from build123d import *

# Parameters (mm, degrees)
SKETCH1_R               = 30
BOSS_EXTRUDE1_DEPTH     = 6
SKETCH2_R               = 14.5
BOSS_EXTRUDE2_DEPTH     = 13
CUT_EXTRUDE1_DEPTH      = 47.486557197
CUT_EXTRUDE1_DEPTH_BACK = 47.486557197
SKETCH3_R               = 12.75
BOSS_EXTRUDE4_START     = 13
SKETCH5_R               = 30
SKETCH5_R_2             = 12.75
BOSS_EXTRUDE4_DEPTH     = 6
CUT_EXTRUDE2_DEPTH      = 45.373415465
CUT_EXTRUDE2_DEPTH_BACK = 45.373415465
SKETCH6_R               = 2
CUT_EXTRUDE3_DEPTH      = 47.486557197
CUT_EXTRUDE3_DEPTH_BACK = 47.486557197
FILLET1_R               = 2
FILLET2_R               = 2
FILLET3_R               = 2
FILLET4_R               = 2
SKETCH8_R               = 4
BOSS_EXTRUDE5_DEPTH     = 13
FILLET5_R               = 2
FILLET6_R               = 2
FILLET7_R               = 2
FILLET8_R               = 2
CUT_EXTRUDE4_DEPTH      = 42.830642507
CUT_EXTRUDE4_DEPTH_BACK = 42.830642507
SKETCH11_W              = 25.5
SKETCH11_H              = 25


with BuildPart() as part:
    # Sketch1 → Boss-Extrude1 (new body)
    with BuildSketch(Plane.XY):
        Circle(SKETCH1_R)
    extrude(amount=-BOSS_EXTRUDE1_DEPTH)

    # Sketch2 → Boss-Extrude2 (add)
    with BuildSketch(Plane.XY):
        with Locations(Location((0, 0, 0), (0, 0, 180))):
            Circle(SKETCH2_R)
    extrude(amount=BOSS_EXTRUDE2_DEPTH)

    # Sketch3 → Cut-Extrude1 (cut, two sides: drawn at the far end of the back side and taken through both)
    with BuildSketch(Plane.XY.offset(13).offset(-CUT_EXTRUDE1_DEPTH_BACK)):
        Circle(SKETCH3_R)
    extrude(amount=CUT_EXTRUDE1_DEPTH + CUT_EXTRUDE1_DEPTH_BACK, mode=Mode.SUBTRACT)

    # Sketch5 → Boss-Extrude4 (add)
    with BuildSketch(Plane.XY.offset(BOSS_EXTRUDE4_START)):
        Circle(SKETCH5_R)
        Circle(SKETCH5_R_2, mode=Mode.SUBTRACT)
    extrude(amount=-BOSS_EXTRUDE4_DEPTH)

    # Sketch6 → Cut-Extrude2 (cut, two sides: drawn at the far end of the back side and taken through both)
    with BuildSketch(Plane.XY.offset(-CUT_EXTRUDE2_DEPTH_BACK)):
        with Locations((-20.333162568, -12.75)):
            Circle(SKETCH6_R)
        with Locations((-22.659159296, 12.75)):
            Circle(SKETCH6_R)
        with Locations((20.333162568, -12.75)):
            Circle(SKETCH6_R)
        with Locations((22.659159296, 12.75)):
            Circle(SKETCH6_R)
    extrude(amount=CUT_EXTRUDE2_DEPTH + CUT_EXTRUDE2_DEPTH_BACK, mode=Mode.SUBTRACT)

    # Sketch7 → Cut-Extrude3 (cut, two sides: drawn at the far end of the back side and taken through both)
    with BuildSketch(Plane.XY.offset(13).offset(-CUT_EXTRUDE3_DEPTH_BACK)):
        with BuildLine():
            Line((10.445298657, -12.448222201), (19.283628291, -22.981333294))
            ThreePointArc((19.283628291, -22.981333294), (0, -30), (-19.283628291, -22.981333294))
            Line((-19.283628291, -22.981333294), (-10.445298657, -12.448222201))
            ThreePointArc((-10.445298657, -12.448222201), (0, -16.25), (10.445298657, -12.448222201))
        make_face()
        with BuildLine():
            Line((-10.445298657, 12.448222201), (-19.283628291, 22.981333294))
            ThreePointArc((-19.283628291, 22.981333294), (0, 30), (19.283628291, 22.981333294))
            Line((19.283628291, 22.981333294), (10.445298657, 12.448222201))
            ThreePointArc((10.445298657, 12.448222201), (0, 16.25), (-10.445298657, 12.448222201))
        make_face()
    extrude(amount=CUT_EXTRUDE3_DEPTH + CUT_EXTRUDE3_DEPTH_BACK, mode=Mode.SUBTRACT)

    # Fillet1
    fillet1_edges = [part.edges().sort_by_distance(p)[0] for p in [
        (-19.283628291, -22.981333294, 10),
    ]]
    fillet(fillet1_edges, radius=FILLET1_R)

    # Fillet2
    fillet2_edges = [part.edges().sort_by_distance(p)[0] for p in [
        (-19.283628291, 22.981333294, 10),
    ]]
    fillet(fillet2_edges, radius=FILLET2_R)

    # Fillet3
    fillet3_edges = [part.edges().sort_by_distance(p)[0] for p in [
        (19.283628291, 22.981333294, 10),
    ]]
    fillet(fillet3_edges, radius=FILLET3_R)

    # Fillet4
    fillet4_edges = [part.edges().sort_by_distance(p)[0] for p in [
        (19.283628291, -22.981333294, 10),
    ]]
    fillet(fillet4_edges, radius=FILLET4_R)

    # Sketch8 → Boss-Extrude5 (add)
    with BuildSketch(Plane.XY.offset(13)):
        with Locations((-22, 0)):
            Circle(SKETCH8_R)
        with Locations((22, 0)):
            Circle(SKETCH8_R)
    extrude(amount=-BOSS_EXTRUDE5_DEPTH)

    # Fillet5
    fillet5_edges = [part.edges().sort_by_distance(p)[0] for p in [
        (-19.283628291, 22.981333294, -3),
    ]]
    fillet(fillet5_edges, radius=FILLET5_R)

    # Fillet6
    fillet6_edges = [part.edges().sort_by_distance(p)[0] for p in [
        (-19.283628291, -22.981333294, -3),
    ]]
    fillet(fillet6_edges, radius=FILLET6_R)

    # Fillet7
    fillet7_edges = [part.edges().sort_by_distance(p)[0] for p in [
        (19.283628291, -22.981333294, -3),
    ]]
    fillet(fillet7_edges, radius=FILLET7_R)

    # Fillet8
    fillet8_edges = [part.edges().sort_by_distance(p)[0] for p in [
        (19.283628291, 22.981333294, -3),
    ]]
    fillet(fillet8_edges, radius=FILLET8_R)

    # Sketch11 → Cut-Extrude4 (cut, two sides: drawn at the far end of the back side and taken through both)
    with BuildSketch(Plane(origin=(0, 0, -6), x_dir=(-1, 0, 0), z_dir=(0, 0, -1)).offset(-CUT_EXTRUDE4_DEPTH_BACK)):
        with Locations((0, 12.5)):
            Rectangle(SKETCH11_W, SKETCH11_H)
    extrude(amount=CUT_EXTRUDE4_DEPTH + CUT_EXTRUDE4_DEPTH_BACK, mode=Mode.SUBTRACT)


solid = part.part
Part model, mm, in its own coordinate system. A direction names the side the tool comes from. Round coordinates to 2 decimals unless told otherwise and drop trailing zeros. Write each loop counter-clockwise with the first axis right and the second up, starting at its lowest first coordinate (ties: lowest second). Pieces come first, ordered by that corner, then holes. Notation, with made-up numbers: M 77,44.5 L 83,44.5 A24 cw 83,56.5 Z; hole C 37.25,74 d10. An arc over 180 degrees is marked long. Return JSON: item names as keys, results as strings. Group by question number.
(1) Pin check, flat tips, straight feed: pin 1 Ø6 at (x, y) = (4, -9) entering from -Z; pin 2 Ø3 at (y, z) = (6.5, -4) entering from -X; pin 3 Ø1.5 at (x, z) = (-2, 6.5) entering from +Y; pin 4 Ø2.5 at (x, y) = (20.33, -12.75) entering from +Z. Stop position of each tip, or through.
(2) Saw through at C-C on y = -3. Write the cut outline in (x, z).
(3) Two-plate mould, pull along Y, no slides. Class faces 5 (the face through (-20.75, 13.35, 9.96)), 6 (the face through (-0.28, -12.747, 3.367)), 7 (the face through (13, 0, 13)): +Y half, -Y half, draft (parallel to the pull), parting line (faces both ways), or undercut.
(4) Drill centre lines: probe 1 along Z at (x, y) = (19, 5.5); probe 2 along X at (y, z) = (-13, -1); probe 3 along Y at (x, z) = (22, 4.25). Where is each one in solid material? Low to high.
(5) Saw through at D-D on x = 0. Write the cut outline in (y, z), then the cut area to 4 significant figures.
(6) Saw through at B-B on z = -3.75. Write the cut outline in (x, y), then the cut area to 3 significant figures.
(7) Which spindle directions (+Z, -Z, +X, -X, +Y, -Y) get a long thin tool onto all of the face, cutting with end or side? Do faces 1 (the face through (-12.75, 6, 4)), 2 (the face through (-14.25, -16.98, -3.04)), 3 (the face through (-14, -5, 7)), 4 (the face through (-30, 0, -3)). Say none if no direction does.
(8) Saw through at A-A on y = 16. Write the cut outline in (x, z).
Returned:
{
 "1": {"pin 1": "z = -6", "pin 2": "x = -29.58", "pin 3": "y = -12.45", "pin 4": "through"},
 "2": {"outline": "M -29.85,-6 L -12.39,-6 L -12.39,13 L -29.85,13 L -29.85,7 L -24.65,7 L -24.65,0 L -29.85,0 Z; M 12.39,-6 L 29.85,-6 L 29.85,0 L 24.65,0 L 24.65,7 L 29.85,7 L 29.85,13 L 12.39,13 Z; hole M -19.35,0 L -14.19,0 L -14.19,7 L -19.35,7 Z; hole M 14.19,0 L 19.35,0 L 19.35,7 L 14.19,7 Z"},
 "3": {"face 5": "undercut", "face 6": "+Y half", "face 7": "draft"},
 "4": {"probe 1": "-6 to 0, 7 to 13", "probe 2": "-27.04 to -22.32, -18.35 to -10.91, -9.75 to 9.75, 10.91 to 18.35, 22.32 to 27.04", "probe 3": "-4 to 4"},
 "5": {"outline": "M -16.25,-6 L -12.75,-6 L -12.75,13 L -16.25,13 L -16.25,7 L -14.5,7 L -14.5,0 L -16.25,0 Z", "area": "54.25 mm²"},
 "6": {"outline": "M -20.88,-21.55 A2 ccw -17.95,-21.39 L -10.45,-12.45 A16.25 ccw 10.45,-12.45 L 17.95,-21.39 A2 ccw 20.88,-21.55 A30 ccw 20.88,21.55 A2 ccw 17.95,21.39 L 12.75,15.19 L 12.75,0 A12.75 cw -12.75,0 L -12.75,15.19 L -17.95,21.39 A2 ccw -20.88,21.55 A30 ccw Z; hole C -22.66,12.75 d4; hole C -20.33,-12.75 d4; hole C 20.33,-12.75 d4; hole C 22.66,12.75 d4", "area": "1,250 mm²"},
 "7": {"face 1": "+Z, -Z, +Y", "face 2": "+Z, -Z, -Y", "face 3": "none", "face 4": "+Z, -Z, -X"},
 "8": {"outline": "M -25.38,-6 L -13.43,-6 L -13.43,0 L -25.38,0 Z; M -25.38,7 L -13.43,7 L -13.43,13 L -25.38,13 Z; M 13.43,-6 L 25.38,-6 L 25.38,0 L 13.43,0 Z; M 13.43,7 L 25.38,7 L 25.38,13 L 13.43,13 Z"}
}
